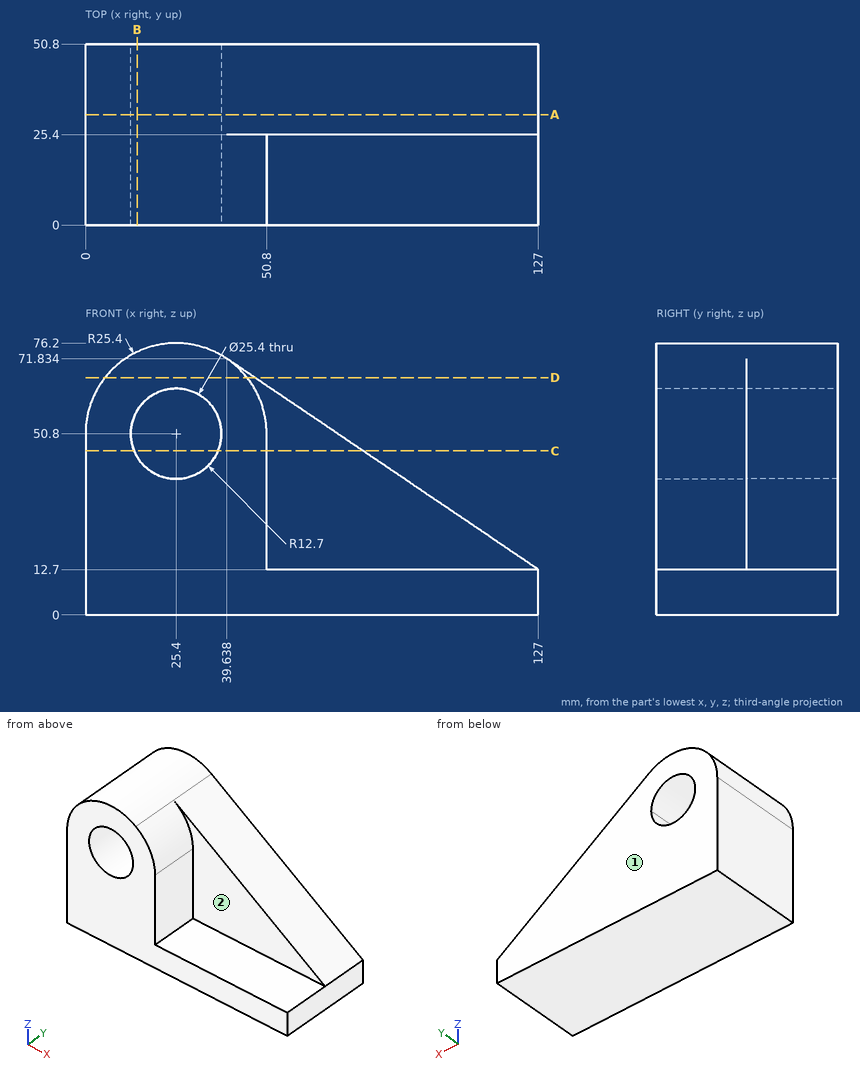
The figure shows three views and two pictorial views of one solid part (mm, origin at its lowest corner). Answer the questions. A direction names the side the tool comes from. Give positions to 0.01 mm unless a question says otherwise; leave off trailing zeros. Order: outer loops, then holes, each group sorted by start corner. A loop starts at its lowest first (then second) coordinate and runs counter-clockwise, first axis right, second up. Notation, with made-up numbers: M 50,0 L 92,0 A8 cw 92,4 Z; hole C 17,59 d6. An arc over 180 degrees is marked long. Return JSON: item names as keys, results as strings.
1) Each of these flat-tipped pins is pushed along its axis until it touches: pin 1 (17.5 mm diameter, centred on x = 103, z = 30, fed in from -Y); pin 2 (20.5 mm diameter, centred on y = 18.5, z = 26.5, fed in from +X); pin 3 (4 mm diameter, centred on x = 97.5, y = 30, fed in from -Z); pin 4 (2 mm diameter, centred on x = 56, y = 21.5, fed in from +Z). Where does it stop, or does it pass through?
Resolved:
{"pin 1": "y = 25.4", "pin 2": "x = 117.81", "pin 3": "z = 0", "pin 4": "z = 12.7"}
2) Section D-D, the plane z = 66.5 is taken. Write down the section's boundary in (x, y).
Resolved:
{"outline": "M 5.43,0 L 45.37,0 L 45.37,25.4 L 47.52,25.4 L 47.52,50.8 L 5.43,50.8 Z"}
3) Straight lines are drawn through the part: line 1 along Z through (x, y) = (25, 17); line 2 along X through (y, z) = (9, 50.8); line 3 along Y through (x, z) = (60, 35.5). For each, find the intervals that lie inside material, in ascending order. Write a range as [from, to].
Resolved:
{"line 1": "[0, 38.11], [63.49, 76.2]", "line 2": "[0, 12.7], [38.1, 50.8]", "line 3": "[25.4, 50.8]"}
4) Section C-C, the plane z = 46 is taken. Write down the section's boundary in (x, y), plus the area to 3 significant figures.
Resolved:
{"outline": "M 0,0 L 13.64,0 L 13.64,50.8 L 0,50.8 Z; M 37.16,0 L 50.8,0 L 50.8,25.4 L 77.8,25.4 L 77.8,50.8 L 37.16,50.8 Z", "area": "2,070 mm^2"}
5) Section B-B, the plane x = 14.5 is taken. Write down the section's boundary in (y, z), plus the area to 3 significant figures.
Resolved:
{"outline": "M 0,0 L 50.8,0 L 50.8,44.28 L 0,44.28 Z; M 0,57.32 L 50.8,57.32 L 50.8,73.74 L 0,73.74 Z", "area": "3,080 mm^2"}
6) Section A-A, the plane y = 31 is taken. Write down the section's boundary in (x, z), plus the area to 3 significant figures.
Resolved:
{"outline": "M 0,0 L 127,0 L 127,12.7 L 39.64,71.83 A25.4 ccw 0,50.8 Z; hole C 25.4,50.8 d25.4", "area": "6,050 mm^2"}
7) A tool of negligible diameter and unlimited length cuts with its end or side. For the marked faces 1 and 2, from which of +Z, -Z, +X, -X, +Y, -Y can it reach the whole face along a straight path? Write none if from no direction.
Resolved:
{"face 1": "+Z, -Z, +X, -X, +Y", "face 2": "+Z, +X, -Y"}
